```python
from build123d import *

# Parameters (mm, degrees)
SKETCH1_W                      = 76.2
SKETCH1_H                      = 25.4
BOSS_EXTRUDE1_DEPTH            = 6.35
SKETCH5_R                      = 12.7
BOSS_EXTRUDE3_DEPTH            = 2.54
SKETCH7_R                      = 20.32
BOSS_EXTRUDE4_DEPTH            = 7.62
SKETCH8_R                      = 15.305053728
CUT_EXTRUDE1_DEPTH             = 2.54
FILLET3_R                      = 2.54
FILLET4_R                      = 2.54
F_97_0_31_DIAMETER_HOLE1_D     = 7.874
F_97_0_31_DIAMETER_HOLE1_DEPTH = 25.4
F_97_0_31_DIAMETER_HOLE1_TIP   = 2.365588257


with BuildPart() as part:
    # Sketch1 → Boss-Extrude1 (new, symmetric)
    with BuildSketch(Plane.XY):
        Rectangle(SKETCH1_W, SKETCH1_H)
    extrude(amount=BOSS_EXTRUDE1_DEPTH, both=True)

    # Sketch5 → Boss-Extrude3 (add)
    with BuildSketch(Plane(origin=(0, 12.7, 0), x_dir=(1, 0, 0), z_dir=(0, 1, 0))):
        with Locations(Location((0, 0, 0), (0, 0, 30))):
            Circle(SKETCH5_R)
    extrude(amount=BOSS_EXTRUDE3_DEPTH)

    # Sketch7 → Boss-Extrude4 (add)
    with BuildSketch(Plane(origin=(0, 15.24, 0), x_dir=(1, 0, 0), z_dir=(0, 1, 0))):
        with Locations(Location((0, 0, 0), (0, 0, 90))):
            Circle(SKETCH7_R)
    extrude(amount=BOSS_EXTRUDE4_DEPTH)

    # Sketch8 → Cut-Extrude1 (cut)
    with BuildSketch(Plane(origin=(0, 22.86, 0), x_dir=(1, 0, 0), z_dir=(0, 1, 0))):
        with Locations(Location((0, 0, 0), (0, 0, 270))):
            Circle(SKETCH8_R)
    extrude(amount=-CUT_EXTRUDE1_DEPTH, mode=Mode.SUBTRACT)

    # Fillet3
    fillet3_edges = [part.edges().sort_by_distance(p)[0] for p in [
        (0, 22.86, 20.32),
    ]]
    fillet(fillet3_edges, radius=FILLET3_R)

    # Fillet4
    fillet4_edges = [part.edges().sort_by_distance(p)[0] for p in [
        (-38.1, 0, 6.35),
        (0, -12.7, 6.35),
        (38.1, 0, 6.35),
        (0, -12.7, -6.35),
        (-38.1, 0, -6.35),
        (38.1, 0, -6.35),
        (38.1, -12.7, 0),
        (-38.1, 12.7, 0),
        (38.1, 12.7, 0),
    ]]
    fillet(fillet4_edges, radius=FILLET4_R)

    # #97 (0.31) Diameter Hole1
    with Locations(Plane.XY.offset(6.35)):
        with Locations((25.4, 0), (-25.4, 0)):
            Hole(F_97_0_31_DIAMETER_HOLE1_D / 2, depth=F_97_0_31_DIAMETER_HOLE1_DEPTH)
            with Locations((0, 0, -(F_97_0_31_DIAMETER_HOLE1_DEPTH + F_97_0_31_DIAMETER_HOLE1_TIP / 2))):  # 118° drill point
                Cone(0, F_97_0_31_DIAMETER_HOLE1_D / 2, F_97_0_31_DIAMETER_HOLE1_TIP, mode=Mode.SUBTRACT)


solid = part.part
```
The listing builds one solid part. Answer for the finished solid, in the listing's coordinates (mm). A direction names the side the tool comes from. Coordinates: 2 decimals unless noted, no trailing zeros. Loops run counter-clockwise (first coordinate to the right, second up) from the corner with the lowest first, then second, coordinate; pieces in that order, holes last. Notation, with made-up numbers: (38, 38) -> (52, 38) arc R15 ccw to (52, 50) -> close; hole circle Ø11 at (45, 54). An arc over 180 degrees is marked (long way). Use one line per item in the form item = value. Start each with the question number.
Item 1: The part is cut by section D-D on x = 0. Determine the outline of the cut face in (y, z).
Item 2: The part is cut by section B-B on y = -5. Determine the outline of the cut face in (x, z), then the cut area to 3 significant figures.
Item 3: A tool of negligible diameter and unlimited length cuts with its end or side. For faces 1 (the face through (-1, 12.7, 9)), 2 (the face through (8.583, 13.952, -9.36)), 3 (the face through (1, 12.7, -9)), from which of +Z, -Z, +X, -X, +Y, -Y can it reach the whole face along a straight path? Write none if from no direction.
Item 4: The mould has two halves that part along X. Classify faces 4 (the face through (0, 20.32, 0)), 5 (the face through (-0.754, -11.936, 5.626)), 6 (the face through (-37.376, 0.178, 5.586)): released by +X, released by -X, zero draft, split by the parting line, or undercut.
Item 5: Flat-ended cylindrical pins translate along their axes: pin 1 Ø4 at (x, z) = (1, 13) entering from +Y; pin 2 Ø4 at (x, z) = (28.5, 1) entering from +Y; pin 3 Ø5 at (x, y) = (-15.5, 0.5) entering from +Z; pin 4 Ø1 at (x, z) = (20.5, 8) entering from +Y. Find the tip coordinate at first contact, or state that the pin passes through.
Item 6: Consider L1, parallel to Y at x = 25.4, z = -2.5; L2, parallel to Y at x = -14.5, z = 2.5; L3, parallel to Z at x = -24, y = 10. Determine where each line is inside the solid, lowest interval first. Write a range as [from, to].
Item 7: The part is cut by section A-A on x = 25.4. Determine the outline of the cut face in (y, z).
Item 8: The part is cut by section C-C on y = 1.5. Determine the outline of the cut face in (x, z), then the cut area to 3 significant figures.
Answer key:
q1.outline = (-12.7, -3.81) arc R2.54 ccw to (-10.16, -6.35) -> (12.7, -6.35) -> (12.7, -12.7) -> (15.24, -12.7) -> (15.24, -20.32) -> (20.32, -20.32) arc R2.54 ccw to (22.86, -17.78) -> (22.86, -15.31) -> (20.32, -15.31) -> (20.32, 15.31) -> (22.86, 15.31) -> (22.86, 17.78) arc R2.54 ccw to (20.32, 20.32) -> (15.24, 20.32) -> (15.24, 12.7) -> (12.7, 12.7) -> (12.7, 6.35) -> (-10.16, 6.35) arc R2.54 ccw to (-12.7, 3.81) -> close
q2.outline = (-38.1, -3.81) arc R2.54 ccw to (-35.56, -6.35) -> (35.56, -6.35) arc R2.54 ccw to (38.1, -3.81) -> (38.1, 3.81) arc R2.54 ccw to (35.56, 6.35) -> (-35.56, 6.35) arc R2.54 ccw to (-38.1, 3.81) -> close
q2.area = 962 mm2
q3.face_1 = +Z, +X, -X, -Y
q3.face_2 = none
q3.face_3 = -Z, +X, -X, -Y
q4.face_4 = undercut
q4.face_5 = zero draft
q4.face_6 = released by -X
q5.pin_1 = 20.32
q5.pin_2 = 12.7
q5.pin_3 = 6.35
q5.pin_4 = through
q6.L1 = [-12.7, -3.94], [3.94, 12.7]
q6.L2 = [-12.7, 12.7], [15.24, 20.32]
q6.L3 = [-6.35, 6.35]
q7.outline = (-12.7, -3.81) arc R2.54 ccw to (-10.16, -6.35) -> (-3.94, -6.35) -> (-3.94, 6.35) -> (-10.16, 6.35) arc R2.54 ccw to (-12.7, 3.81) -> close; (3.94, -6.35) -> (12.7, -6.35) -> (12.7, 6.35) -> (3.94, 6.35) -> close
q8.outline = (-38.1, -3.81) arc R2.54 ccw to (-35.56, -6.35) -> (-29.04, -6.35) -> (-29.04, 6.35) -> (-35.56, 6.35) arc R2.54 ccw to (-38.1, 3.81) -> close; (-21.76, -6.35) -> (21.76, -6.35) -> (21.76, 6.35) -> (-21.76, 6.35) -> close; (29.04, -6.35) -> (35.56, -6.35) arc R2.54 ccw to (38.1, -3.81) -> (38.1, 3.81) arc R2.54 ccw to (35.56, 6.35) -> (29.04, 6.35) -> close
q8.area = 777 mm2
